The listing builds one solid part. Answer for the finished solid, in the listing's coordinates (mm). Give positions to 0.01 mm unless a question says otherwise; leave off trailing zeros. Write each loop counter-clockwise with the first axis right and the second up, starting at its lowest first coordinate (ties: lowest second). Pieces come first, ordered by that corner, then holes. Notation, with made-up numbers: (76.25, -35) -> (126.25, -35) arc R24 ccw to (126.25, -17) -> close; hole circle Ø5 at (-1.75, 71.25). An arc over 180 degrees is marked (long way). One line per question, with ' | ' between items.
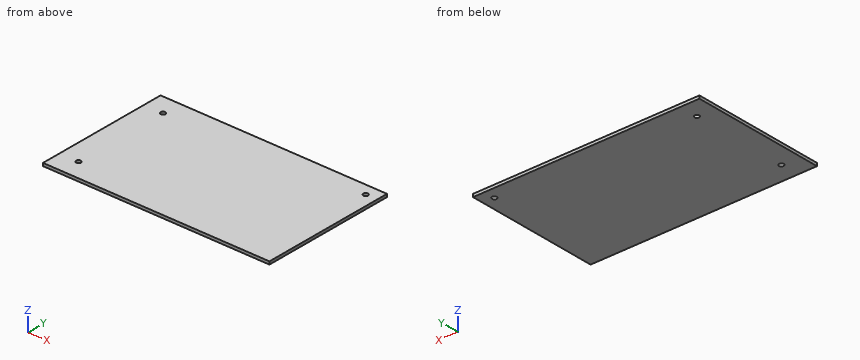
Autodesk Inventor part; units mm, degrees
ref_plane "YZ Plane" through (0, 0, 0) normal (1, 0, 0) x (0, 1, 0)
ref_plane "XZ Plane" through (0, 0, 0) normal (0, 1, 0) x (-1, 0, 0)
ref_plane "XY Plane" through (0, 0, 0) normal (0, 0, 1) x (1, 0, 0)
sketch "Schizzo1" plane through (0, 0, 0) normal (0, 0, 1) x (1, 0, 0)
  line L0 (-59.5, -35.5) -> (59.5, -35.5)
  line L1 (59.5, -35.5) -> (59.5, 35.5)
  line L2 (59.5, 35.5) -> (-59.5, 35.5)
  line L3 (-59.5, 35.5) -> (-59.5, -35.5)
  line L4 (-59.5, -35.5) -> (59.5, 35.5) construction
  line L5 (59.5, -35.5) -> (-59.5, 35.5) construction
  point P0 (0, 0)
  dimension "d0" = 119
  dimension "d1" = 71
extrude "Estrusione1" add sketch "Schizzo1" along normal blind 1.5
sketch "Schizzo4" plane through (0, 0, 1.5) normal (0, 0, 1) x (1, 0, 0)
  line L0 (59.5, 35.5) -> (-59.5, 35.5)
  line L1 (59.5, -35.5) -> (59.5, 35.5)
  line L2 (-59.5, -35.5) -> (59.5, -35.5)
  circle A0 centre (-49.5, 25.5) radius 1.25
  circle A1 centre (-49.5, -25.5) radius 1.25
  line L3 (-59.5, 35.5) -> (-59.5, -35.5)
  circle A2 centre (53.5, 29.5) radius 1.25
  point P0 (0, 0)
  dimension "d17" = 2.5
  dimension "d18" = 2.5
  dimension "d19" = 10
  dimension "d20" = 10
  dimension "d21" = 10
  dimension "d22" = 10
  dimension "d24" = 2.5
  dimension "d27" = 6
  dimension "d28" = 6
extrude "Estrusione3" cut sketch "Schizzo4" against normal blind 1.5 contours A0 | A1 | A2
properties part number "PCB"
Item 1: Find section C-C (x = 53.5). Write down the section's boundary in (y, z), then the cut area to 3 significant figures.
Answers below:
outline: (-35.5, 0) -> (28.25, 0) -> (28.25, 1.5) -> (-35.5, 1.5) -> close; (30.75, 0) -> (35.5, 0) -> (35.5, 1.5) -> (30.75, 1.5) -> close | area: 103 mm²
Item 2: Find section B-B (x = -49.5). Write down the section's boundary in (y, z), then the cut area to 3 significant figures.
Answers below:
outline: (-35.5, 0) -> (-26.75, 0) -> (-26.75, 1.5) -> (-35.5, 1.5) -> close; (-24.25, 0) -> (24.25, 0) -> (24.25, 1.5) -> (-24.25, 1.5) -> close; (26.75, 0) -> (35.5, 0) -> (35.5, 1.5) -> (26.75, 1.5) -> close | area: 99.0 mm²
Item 3: Consider line 1 (Y direction, x = -49.5, z = 0.3). Determine where the line is inside the solid, lowest interval first. Write a range as [from, to].
Answers below:
line 1: [-35.5, -26.75], [-24.25, 24.25], [26.75, 35.5]
Item 4: Find section A-A (y = 25.5). Write down the section's boundary in (x, z).
Answers below:
outline: (-59.5, 0) -> (-50.75, 0) -> (-50.75, 1.5) -> (-59.5, 1.5) -> close; (-48.25, 0) -> (59.5, 0) -> (59.5, 1.5) -> (-48.25, 1.5) -> close
